```python
from build123d import *

# Parameters (mm, degrees)
SKETCH1_W       = 60
SKETCH1_H       = 40
EXTRUDE1_DEPTH  = 3
SKETCH2_W       = 3
SKETCH2_H       = 40
EXTRUDE2_DEPTH  = 14
SKETCH4_R       = 1.5
EXTRUDE3_DEPTH  = 15
SKETCH5_W       = 57
SKETCH5_H       = 14
EXTRUDE4_DEPTH  = 3
SKETCH6_W       = 57
SKETCH6_H       = 14
EXTRUDE5_DEPTH  = 3
SKETCH7_R       = 1.5
EXTRUDE6_DEPTH  = 3
SKETCH8_R       = 2.5
EXTRUDE7_DEPTH  = 3
SKETCH9_W       = 40
SKETCH9_H       = 17
EXTRUDE8_DEPTH  = 3
EXTRUDE9_DEPTH  = 63
EXTRUDE10_DEPTH = 3
EXTRUDE11_DEPTH = 3
EXTRUDE12_DEPTH = 3
EXTRUDE13_DEPTH = 3
SKETCH15_W      = 160
SKETCH15_H      = 100
EXTRUDE14_DEPTH = 5
EXTRUDE15_DEPTH = 5
EXTRUDE16_DEPTH = 5
SKETCH18_W      = 40
SKETCH18_H      = 100
EXTRUDE17_DEPTH = 2
SKETCH19_W      = 10
SKETCH19_H      = 10
EXTRUDE18_DEPTH = 5


with BuildPart() as part:
    # Sketch1 → Extrude1 (new body)
    with BuildSketch(Plane(origin=(0, 0, 0), x_dir=(1, 0, 0), z_dir=(0, 1, 0))):
        Rectangle(SKETCH1_W, SKETCH1_H)
    extrude(amount=EXTRUDE1_DEPTH)

    # Sketch2 → Extrude2 (add)
    with BuildSketch(Plane(origin=(0, 3, 0), x_dir=(1, 0, 0), z_dir=(0, 1, 0))):
        with Locations((28.5, 0)):
            Rectangle(SKETCH2_W, SKETCH2_H)
    extrude(amount=EXTRUDE2_DEPTH)

    # Sketch4 → Extrude3 (cut)
    with BuildSketch(Plane.ZY.offset(-27)):
        with Locations((-12, 10.5)):
            Circle(SKETCH4_R)
        with Locations((12, 10.5)):
            Circle(SKETCH4_R)
    extrude(amount=-EXTRUDE3_DEPTH, mode=Mode.SUBTRACT)

    # Sketch5 → Extrude4 (add)
    with BuildSketch(Plane(origin=(0, 0, -20), x_dir=(-1, 0, 0), z_dir=(0, 0, -1))):
        with Locations((1.5, 10)):
            Rectangle(SKETCH5_W, SKETCH5_H)
    extrude(amount=-EXTRUDE4_DEPTH)

    # Sketch6 → Extrude5 (add)
    with BuildSketch(Plane.XY.offset(20)):
        with Locations((-1.5, 10)):
            Rectangle(SKETCH6_W, SKETCH6_H)
    extrude(amount=-EXTRUDE5_DEPTH)

    # Sketch7 → Extrude6 (cut)
    with BuildSketch(Plane(origin=(0, 3, 0), x_dir=(1, 0, 0), z_dir=(0, 1, 0))):
        with Locations(Location((-5, 10, 0), (0, 0, 270))):
            Circle(SKETCH7_R)
        with Locations(Location((-25, 10, 0), (0, 0, 270))):
            Circle(SKETCH7_R)
        with Locations(Location((-25, -10, 0), (0, 0, 270))):
            Circle(SKETCH7_R)
        with Locations(Location((-5, -10, 0), (0, 0, 270))):
            Circle(SKETCH7_R)
    extrude(amount=-EXTRUDE6_DEPTH, mode=Mode.SUBTRACT)

    # Sketch8 → Extrude7 (cut)
    with BuildSketch(Plane(origin=(0, 3, 0), x_dir=(1, 0, 0), z_dir=(0, 1, 0))):
        with Locations(Location((-15, 0, 0), (0, 0, 270))):
            Circle(SKETCH8_R)
    extrude(amount=-EXTRUDE7_DEPTH, mode=Mode.SUBTRACT)

    # Sketch9 → Extrude8 (add)
    with BuildSketch(Plane.ZY.offset(30)):
        with Locations((0, 8.5)):
            Rectangle(SKETCH9_W, SKETCH9_H)
    extrude(amount=EXTRUDE8_DEPTH)

    # Sketch10 → Extrude9 (add)
    with BuildSketch(Plane(origin=(0, 17, 0), x_dir=(1, 0, 0), z_dir=(0, 1, 0))):
        Polygon((-30, -17), (-30, 17), (2, 17), (2, 20), (-33, 20), (-33, -20), (2, -20), (2, -17), align=None)
    extrude(amount=EXTRUDE9_DEPTH)

    # Mirror2: part across plane


with BuildPart() as part_1:
    add(part.part)
    add(part.part.mirror(Plane.ZX.offset(80)))

    # Sketch11 → Extrude10 (add)
    with BuildSketch(Plane.XY.offset(20)):
        Polygon((-33, 0), (30, 0), (30, 17), (2, 17), (2, 143), (30, 143), (30, 160), (-33, 160), align=None)
    extrude(amount=EXTRUDE10_DEPTH)

    # Sketch12 → Extrude11 (add)
    with BuildSketch(Plane(origin=(0, 0, -20), x_dir=(-1, 0, 0), z_dir=(0, 0, -1))):
        Polygon((-30, 0), (33, 0), (33, 160), (-30, 160), (-30, 143), (-2, 143), (-2, 17), (-30, 17), align=None)
    extrude(amount=EXTRUDE11_DEPTH)

    # Sketch13 → Extrude12 (cut)
    with BuildSketch(Plane(origin=(0, 0, 17), x_dir=(-1, 0, 0), z_dir=(0, 0, -1))):
        Polygon((-27, 17), (-27, 3), (30, 3), (30, 157), (-27, 157), (-27, 143), (-2, 143), (-2, 17), align=None)
    extrude(amount=-EXTRUDE12_DEPTH, mode=Mode.SUBTRACT)

    # Sketch14 → Extrude13 (cut)
    with BuildSketch(Plane.XY.offset(-17)):
        Polygon((27, 17), (2, 17), (2, 143), (27, 143), (27, 157), (-30, 157), (-30, 3), (27, 3), align=None)
    extrude(amount=-EXTRUDE13_DEPTH, mode=Mode.SUBTRACT)

    # Sketch15 → Extrude14 (add)
    with BuildSketch(Plane.ZY.offset(33)):
        with Locations((0, 80)):
            Rectangle(SKETCH15_W, SKETCH15_H)
    extrude(amount=-EXTRUDE14_DEPTH)

    # Sketch16 → Extrude15 (add)
    with BuildSketch(Plane.XZ.offset(-30)):
        Polygon((-28, -23), (2, -23), (-28, -80), align=None)
        Polygon((-28, 23), (2, 23), (-28, 80), align=None)
    extrude(amount=-EXTRUDE15_DEPTH)

    # Sketch17 → Extrude16 (add)
    with BuildSketch(Plane(origin=(0, 130, 0), x_dir=(1, 0, 0), z_dir=(0, 1, 0))):
        Polygon((-28, 80), (-28, 23), (2, 23), align=None)
        Polygon((-28, -23), (-28, -80), (2, -23), align=None)
    extrude(amount=-EXTRUDE16_DEPTH)

    # Sketch18 → Extrude17 (cut)
    with BuildSketch(Plane(origin=(-28, 0, 0), x_dir=(0, 0, -1), z_dir=(1, 0, 0))):
        with Locations((0, 80)):
            Rectangle(SKETCH18_W, SKETCH18_H)
    extrude(amount=-EXTRUDE17_DEPTH, mode=Mode.SUBTRACT)

    # Sketch19 → Extrude18 (cut)
    with BuildSketch(Plane(origin=(30, 0, 0), x_dir=(0, 0, -1), z_dir=(1, 0, 0))):
        with Locations((0, 143)):
            Rectangle(SKETCH19_W, SKETCH19_H)
    extrude(amount=-EXTRUDE18_DEPTH, mode=Mode.SUBTRACT)


solid = part_1.part
```
Work out the finished part from the listing and answer in its coordinate system (mm). A direction names the side the tool comes from. Coordinates: 2 decimals unless noted, no trailing zeros. Loops run counter-clockwise (first coordinate to the right, second up) from the corner with the lowest first, then second, coordinate; pieces in that order, holes last. Notation, with made-up numbers: M 58,66 L 76,66 A14 cw 76,86 Z; hole C 87.5,10 d2. An arc over 180 degrees is marked long. Use CSV: the item, a comma, the result in double quotes. Start each with the question number.
(1) For faces 1 (the face through (21, 143, -21)), 2 (the face through (-17, 125, 45)), 3 (the face through (-30, 81, 0)), 4 (the face through (-9, 12, 23)), determine the directions among +Z, -Z, +X, -X, +Y, -Y from which every point of the face is accessible in a straight line to the end or side of a thin tool.
(2) Find section D-D, the plane z = -56. Give the vertices of the cut face in (x, y).
(3) Find section B-B, the plane z = 38.5. Give the vertices of the cut face in (x, y), then the cut area to 3 significant figures.
(4) For a pull along Y with two mould halves and no side action, classify faces 5 (the face through (-20, 30, 45)), 6 (the face through (-8, 12, -23)), 7 (the face through (20, 143, 21)) as +Y half, -Y half, draft (parallel to the pull), parting line (faces both ways), or undercut.
(5) Consider line 1 (Y direction, x = 28, z = -12); line 2 (Z direction, x = -1.5, y = 55); line 3 (X direction, y = 158, z = -10). Determine where each line is inside the solid, lowest interval first.
(6) Given pin 1 Ø5 at (y, z) = (103, -10.5) entering from +X; pin 2 Ø2.5 at (x, z) = (-5, -10) entering from +Y; pin 3 Ø6 at (x, z) = (-15, 0) entering from -Y; pin 4 Ø9 at (x, z) = (-16, 47.5) entering from +Y, each flat-ended and moving along its own axis, determine where each tip first touches the part or whether it passes through.
(7) Find section A-A, the plane x = 6. Give the vertices of the cut face in (y, z), then the cut area to 3 significant figures.
(8) Find section C-C, the plane y = 56. Give the vertices of the cut face in (x, z).
Recorded:
1,face 1,"+Z, -Z, +X"
1,face 2,"+Z, +X"
1,face 3,"none"
1,face 4,"+Z, +X, -X, -Y"
2,outline,"M -33,30 L -15.37,30 L -15.37,35 L -28,35 L -28,125 L -15.37,125 L -15.37,130 L -33,130 Z"
3,outline,"M -33,30 L -6.16,30 L -6.16,35 L -28,35 L -28,125 L -6.16,125 L -6.16,130 L -33,130 Z"
3,area,"718 mm^2"
4,face 5,"-Y half"
4,face 6,"draft"
4,face 7,"undercut"
5,line 1,"y = 0 to 9, 12 to 17, 143 to 148, 151 to 160"
5,line 2,"z = -23 to -20, 20 to 23"
5,line 3,"x = -33 to -26.5, -23.5 to -6.5, -3.5 to 30"
6,pin 1,"stops at x = -30"
6,pin 2,"passes through"
6,pin 3,"stops at y = 0"
6,pin 4,"stops at y = 130"
7,outline,"M 0,-23 L 17,-23 L 17,-20 L 3,-20 L 3,20 L 17,20 L 17,23 L 0,23 Z; M 143,-23 L 160,-23 L 160,23 L 143,23 L 143,20 L 157,20 L 157,-20 L 143,-20 Z"
7,area,"444 mm^2"
8,outline,"M -33,-80 L -28,-80 L -28,-23 L 2,-23 L 2,-20 L -30,-20 L -30,20 L 2,20 L 2,23 L -28,23 L -28,80 L -33,80 Z"
